Source: CAD feature listing. Evaluate the final solid. Frame: model axes, mm. A direction names the side the tool comes from. Give positions to 0.01 mm unless a question says otherwise; leave off trailing zeros. Answer in a Markdown table with one row per item. Add a question column.
(1) Pin query (flat end, axial travel): P1, Ø6, axis at x = -102.5, y = 21, coming from the -Z side; P2, Ø16, axis at y = 16, z = 125.5, coming from the +X side; P3, Ø4, axis at x = 106.5, y = 10.5, coming from the -Z side. Return the tip coordinate at first contact, or that it passes through.
(2) Section query A-A, the plane x = 69. Count the separate pieces of the cut face and the enclosed holes in it, plus the area to 3 significant figures.
(3) Mould query, pull axis Z, two halves, no side actions, for faces 1 (the face through (50, 30, -3)), 2 (the face through (-233, 2.5, 30.6)), 3 (the face through (121, 35, -190)). Classes: pulls with the +Z half, pulls with the -Z half, needs draft (parallel to the pull), parting line crosses it, or undercut.
(4) Material intervals for line 1 along X through (y, z) = (10.5, -156.5); line 2 along X through (y, z) = (27, -130.5); line 3 along X through (y, z) = (20.5, -35.5), sorted ascending.
(5) Set-up query: faces 4 (the face through (121, 5, 190)), 5 (the face through (-97.181, 19.86, 165.514)). Return all of +Z, -Z, +X, -X, +Y, -Y with unobstructed straight access to the full face (end or side cutting, diameter ignored); none if empty.
from build123d import *

# Parameters (mm, degrees)
CUT_EXTRUDE1_DEPTH = 335.738704066
SKETCH3_R          = 210
CUT_EXTRUDE2_DEPTH = 10
CUT_EXTRUDE3_START = -10
SKETCH4_R          = 210
CUT_EXTRUDE3_DEPTH = 10
CUT_EXTRUDE4_DEPTH = 334.691474269


with BuildPart() as part:
    # Sketch1 → Revolve1 (revolve)
    with BuildSketch(Plane(origin=(0, 0, 0), x_dir=(0, 0, -1), z_dir=(1, 0, 0))):
        Polygon((20, 0), (20, 40), (235, 40), (235, 35), (225, 35), (225, 25), (235, 25), (235, 15), (225, 15), (225, 5), (235, 5), (235, 0), align=None)
    revolve(axis=Axis((0, 0, 0), (0, 1, 0)))

    # Sketch2 → Cut-Extrude1 (cut, through all)
    with BuildSketch(Plane(origin=(0, 40, 0), x_dir=(1, 0, 0), z_dir=(0, 1, 0))):
        with BuildLine():
            Line((-19.995175711, -0.439258804), (-24.04880088, 0.738360519))
            Line((-24.04880088, 0.738360519), (-20.701084967, 12.261936274))
            Line((-20.701084967, 12.261936274), (-16.647459798, 11.084316951))
            ThreePointArc((-16.647459798, 11.084316951), (19.205959591, -5.579526521), (-19.995175711, -0.439258804))
        make_face()
    extrude(amount=-CUT_EXTRUDE1_DEPTH, mode=Mode.SUBTRACT)

    # Sketch3 → Cut-Extrude2 (cut)
    with BuildSketch(Plane(origin=(0, 40, 0), x_dir=(1, 0, 0), z_dir=(0, 1, 0))):
        with Locations(Location((0, 0, 0), (0, 0, 270))):
            Circle(SKETCH3_R)
    extrude(amount=-CUT_EXTRUDE2_DEPTH, mode=Mode.SUBTRACT)

    # Sketch4 → Cut-Extrude3 (cut)
    with BuildSketch(Plane.XZ.offset(CUT_EXTRUDE3_START)):
        with Locations(Location((0, 0, 0), (0, 0, 90))):
            Circle(SKETCH4_R)
    extrude(amount=CUT_EXTRUDE3_DEPTH, mode=Mode.SUBTRACT)

    # Sketch5 → Cut-Extrude4 (cut, through all)
    with BuildSketch(Plane.XZ.offset(-10)):
        with BuildLine():
            Line((0, 43.874821937), (0, 184.699253674))
            ThreePointArc((0, 184.699253674), (3.122729064, 191.958946813), (10.540628894, 194.684629))
            ThreePointArc((10.540628894, 194.684629), (51.279766456, 188.105276849), (89.721606346, 173.098939861))
            ThreePointArc((89.721606346, 173.098939861), (94.717809879, 167.027457013), (93.78003887, 159.220694609))
            Line((93.78003887, 159.220694609), (23.495497372, 37.484297749))
            ThreePointArc((23.495497372, 37.484297749), (18.316966013, 33.109992057), (11.538522594, 33.043342693))
            ThreePointArc((11.538522594, 33.043342693), (9.673276888, 33.636701893), (7.777777778, 34.124861507))
            ThreePointArc((7.777777778, 34.124861507), (2.1826404, 37.638726292), (0, 43.874821937))
        make_face()
        with BuildLine():
            Line((44.21010278, -1.605548725), (184.779185774, -1.605548725))
            ThreePointArc((184.779185774, -1.605548725), (192.008925843, 1.485698961), (194.768882461, 8.848279566))
            ThreePointArc((194.768882461, 8.848279566), (188.543831565, 49.643057974), (173.872148887, 88.213862106))
            ThreePointArc((173.872148887, 88.213862106), (167.802688955, 93.275110708), (159.954245742, 92.349626837))
            Line((159.954245742, 92.349626837), (37.996710384, 21.937410968))
            ThreePointArc((37.996710384, 21.937410968), (33.687413335, 16.929141112), (33.441885854, 10.326677613))
            ThreePointArc((33.441885854, 10.326677613), (33.966876783, 8.441047424), (34.385635495, 6.529017659))
            ThreePointArc((34.385635495, 6.529017659), (37.832577247, 0.692038141), (44.21010278, -1.605548725))
        make_face()
        with BuildLine():
            Line((20.714605407, -39.089846473), (90.999146905, -160.826243334))
            ThreePointArc((90.999146905, -160.826243334), (97.291115964, -165.541758053), (105.047276114, -164.250660295))
            ThreePointArc((105.047276114, -164.250660295), (137.264065109, -138.462218875), (163.331519993, -106.470766894))
            ThreePointArc((163.331519993, -106.470766894), (164.679959892, -98.683836105), (159.954245742, -92.349626837))
            Line((159.954245742, -92.349626837), (37.996710384, -21.937410968))
            ThreePointArc((37.996710384, -21.937410968), (31.504772935, -20.70958518), (25.664108076, -23.798183894))
            ThreePointArc((25.664108076, -23.798183894), (24.293599895, -25.195654469), (22.847112902, -26.514325035))
            ThreePointArc((22.847112902, -26.514325035), (19.515611235, -32.417953916), (20.714605407, -39.089846473))
        make_face()
        with BuildLine():
            Line((-23.495497372, -37.484297749), (-93.78003887, -159.220694609))
            ThreePointArc((-93.78003887, -159.220694609), (-94.717809879, -167.027457013), (-89.721606346, -173.098939861))
            ThreePointArc((-89.721606346, -173.098939861), (-51.279766456, -188.105276849), (-10.540628894, -194.684629))
            ThreePointArc((-10.540628894, -194.684629), (-3.122729064, -191.958946813), (0, -184.699253674))
            Line((0, -184.699253674), (0, -43.874821937))
            ThreePointArc((0, -43.874821937), (-2.1826404, -37.638726292), (-7.777777778, -34.124861507))
            ThreePointArc((-7.777777778, -34.124861507), (-9.673276888, -33.636701893), (-11.538522594, -33.043342693))
            ThreePointArc((-11.538522594, -33.043342693), (-18.316966013, -33.109992057), (-23.495497372, -37.484297749))
        make_face()
        with BuildLine():
            Line((-44.21010278, 1.605548725), (-184.779185774, 1.605548725))
            ThreePointArc((-184.779185774, 1.605548725), (-192.008925843, -1.485698961), (-194.768882461, -8.848279566))
            ThreePointArc((-194.768882461, -8.848279566), (-188.543831565, -49.643057974), (-173.872148887, -88.213862106))
            ThreePointArc((-173.872148887, -88.213862106), (-167.802688955, -93.275110708), (-159.954245742, -92.349626837))
            Line((-159.954245742, -92.349626837), (-37.996710384, -21.937410968))
            ThreePointArc((-37.996710384, -21.937410968), (-33.687413335, -16.929141112), (-33.441885854, -10.326677613))
            ThreePointArc((-33.441885854, -10.326677613), (-33.966876783, -8.441047424), (-34.385635495, -6.529017659))
            ThreePointArc((-34.385635495, -6.529017659), (-37.832577247, -0.692038141), (-44.21010278, 1.605548725))
        make_face()
        with BuildLine():
            Line((-20.714605407, 39.089846473), (-90.999146905, 160.826243334))
            ThreePointArc((-90.999146905, 160.826243334), (-97.291115964, 165.541758053), (-105.047276114, 164.250660295))
            ThreePointArc((-105.047276114, 164.250660295), (-137.264065109, 138.462218875), (-163.331519993, 106.470766894))
            ThreePointArc((-163.331519993, 106.470766894), (-164.679959892, 98.683836105), (-159.954245742, 92.349626837))
            Line((-159.954245742, 92.349626837), (-37.996710384, 21.937410968))
            ThreePointArc((-37.996710384, 21.937410968), (-31.504772935, 20.70958518), (-25.664108076, 23.798183894))
            ThreePointArc((-25.664108076, 23.798183894), (-24.293599895, 25.195654469), (-22.847112902, 26.514325035))
            ThreePointArc((-22.847112902, 26.514325035), (-19.515611235, 32.417953916), (-20.714605407, 39.089846473))
        make_face()
    extrude(amount=-CUT_EXTRUDE4_DEPTH, mode=Mode.SUBTRACT)


solid = part.part
Values follow:
| question | item | result |
|---|---|---|
| 1 | P1 | stops at z = -212.9 |
| 1 | P2 | stops at x = 203.52 |
| 1 | P3 | stops at z = -199.26 |
| 2 | separate pieces | 4 |
| 2 | enclosed holes | 0 |
| 2 | area | 5,810 mm² |
| 3 | face 1 | undercut |
| 3 | face 2 | parting line crosses it |
| 3 | face 3 | needs draft |
| 4 | line 1 | x = -161.66 to -92.21, 0 to 88.5, 116.28 to 161.66 |
| 4 | line 2 | x = -183.29 to -77.2, 0 to 73.49, 144.85 to 183.29 |
| 4 | line 3 | x = -232.3 to -191.71, -61.49 to -21.99, -4.54 to 19.47, 61.49 to 232.3 |
| 5 | face 4 | none |
| 5 | face 5 | +Y, -Y |
